```python
from build123d import *

# Parameters (mm, degrees)
F1_DEPTH = 2
F2_W     = 16.5
F2_H     = 16.5
F3_DEPTH = 25
F4_W     = 14.5
F4_H     = 14.5
F5_DEPTH = 24


with BuildPart() as f1:
    # F0 (on Top) → F1 (new body)
    with BuildSketch(Plane.XY):
        Polygon((10, -10), (-10, 10), (-10, -10), align=None)
        Polygon((10, 10), (-10, 10), (10, -10), align=None)
    extrude(amount=F1_DEPTH)

    # F2 (on face) → F3 (join)
    with BuildSketch(Plane.XY.offset(2)):
        Rectangle(F2_W, F2_H)
    extrude(amount=F3_DEPTH)

    # F4 (on face) → F5 (cut)
    with BuildSketch(Plane.XY.offset(27)):
        Rectangle(F4_W, F4_H)
    extrude(amount=-F5_DEPTH, mode=Mode.SUBTRACT)


solid = f1.part
```
The listing builds one solid part. Answer for the finished solid, in the listing's coordinates (mm). A direction names the side the tool comes from. Round coordinates to 2 decimals unless told otherwise and drop trailing zeros. Loops run counter-clockwise (first coordinate to the right, second up) from the corner with the lowest first, then second, coordinate; pieces in that order, holes last. Notation, with made-up numbers: (-35, 20.25) - (-27, 20.25) arc R17 cw to (-27, 42.25) - close; hole circle Ø1 at (66, 57.25). An arc over 180 degrees is marked (long way). Return JSON: item names as keys, results as strings. Group by question number.
1. The mould has two halves that part along X. Classify faces 6 (the flat face through (0, -7.25, 15)), 7 (the flat face through (8.25, 0, 14)), 8 (the flat face through (0, -8.25, 14)): pulls with the +X half, pulls with the -X half, needs draft (parallel to the pull), parting line crosses it, or undercut.
2. Consider probe 1 along X at (y, z) = (5.5, 3.75); probe 2 along Z at (x, y) = (4.75, 0). Determine where each line is inside the solid, lowest interval first.
3. Each of these flat-tipped pins is pushed along its axis until it touches: P1, Ø6, axis at y = 4, z = 19.5, coming from the -X side; P2, Ø4, axis at x = 1.5, y = 3, coming from the +Z side; P3, Ø4.5, axis at x = 1.5, z = 18, coming from the -Y side. Where does it stop, or does it pass through?
4. The part is cut by section B-B on x = -7.75. Determine the outline of the cut face in (y, z), then the cut area to 4 significant figures.
5. The part is cut by section C-C on y = 2.25. Determine the outline of the cut face in (x, z).
6. The part is cut by section A-A on z = 17.5. Determine the outline of the cut face in (x, y).
7. The part is cut by section D-D on z = 2.5. Determine the outline of the cut face in (x, y), then the cut area to 3 significant figures.
8. Which of the six approach directions +Z, -Z, +X, -X, +Y, -Y give full straight-line access (tool end or side, diameter ignored) to faces 1 (the flat face through (0, 10, 1)), 2 (the flat face through (7.25, 0, 15)), 3 (the flat face through (0, 8.25, 14)), 4 (the flat face through (0, -10, 1)), 5 (the flat face through (-8.25, 0, 14))?
Resolved:
{
 "1": {"face 6": "undercut", "face 7": "pulls with the +X half", "face 8": "needs draft"},
 "2": {"probe 1": "x = -8.25 to -7.25, 7.25 to 8.25", "probe 2": "z = 0 to 3"},
 "3": {"P1": "stops at x = -8.25", "P2": "stops at z = 3", "P3": "stops at y = -8.25"},
 "4": {"outline": "(-10, 0) - (10, 0) - (10, 2) - (8.25, 2) - (8.25, 27) - (-8.25, 27) - (-8.25, 2) - (-10, 2) - close", "area": "452.5 mm²"},
 "5": {"outline": "(-10, 0) - (10, 0) - (10, 2) - (8.25, 2) - (8.25, 27) - (7.25, 27) - (7.25, 3) - (-7.25, 3) - (-7.25, 27) - (-8.25, 27) - (-8.25, 2) - (-10, 2) - close"},
 "6": {"outline": "(-8.25, -8.25) - (8.25, -8.25) - (8.25, 8.25) - (-8.25, 8.25) - close; hole (-7.25, -7.25) - (7.25, -7.25) - (7.25, 7.25) - (-7.25, 7.25) - close"},
 "7": {"outline": "(-8.25, -8.25) - (8.25, -8.25) - (8.25, 8.25) - (-8.25, 8.25) - close", "area": "272 mm²"},
 "8": {"face 1": "+Z, -Z, +X, -X, +Y", "face 2": "+Z", "face 3": "+Z, +X, -X, +Y", "face 4": "+Z, -Z, +X, -X, -Y", "face 5": "+Z, -X, +Y, -Y"}
}
